from build123d import *

# Parameters (mm, degrees)
SKETCH3_W           = 30
SKETCH3_H           = 30
BOSS_EXTRUDE2_DEPTH = 5
SKETCH4_W           = 22
SKETCH4_H           = 22
BOSS_EXTRUDE3_DEPTH = 3
SKETCH10_R          = 1.5
CUT_EXTRUDE2_DEPTH  = 23.671568098
BOSS_EXTRUDE4_DEPTH = 2.5
SKETCH13_W          = 20
SKETCH13_H          = 3
BOSS_EXTRUDE6_DEPTH = 7.5
FILLET1_R           = 5
MIRROR2_START       = 223.674571743
MIRROR2_OUTLINE_W   = 20
MIRROR2_OUTLINE_H   = 15
MIRROR2_DEPTH       = 3
FILLET2_R           = 5


# Read off the part's stored shape, not the designer's step: Loft-Thin2, Mirror2
with BuildPart() as part:
    # Sketch3 → Boss-Extrude2 (new body)
    with BuildSketch(Plane(origin=(0, 0, 0), x_dir=(1, 0, 0), z_dir=(0, 1, 0))):
        Rectangle(SKETCH3_W, SKETCH3_H)
    extrude(amount=BOSS_EXTRUDE2_DEPTH)

    # Sketch4 → Boss-Extrude3 (add)
    with BuildSketch(Plane(origin=(0, 5, 0), x_dir=(1, 0, 0), z_dir=(0, 1, 0))):
        Rectangle(SKETCH4_W, SKETCH4_H)
    extrude(amount=BOSS_EXTRUDE3_DEPTH)

    # Sketch10 → Cut-Extrude2 (cut, through all)
    with BuildSketch(Plane(origin=(0, 8, 0), x_dir=(1, 0, 0), z_dir=(0, 1, 0))):
        with Locations(Location((-7.071067812, -7.071067812, 0), (0, 0, 270))):
            Circle(SKETCH10_R)
        with Locations(Location((-7.071067812, 7.071067812, 0), (0, 0, 270))):
            Circle(SKETCH10_R)
        with Locations(Location((7.071067812, 7.071067812, 0), (0, 0, 270))):
            Circle(SKETCH10_R)
        with Locations(Location((7.071067812, -7.071067812, 0), (0, 0, 270))):
            Circle(SKETCH10_R)
    extrude(amount=-CUT_EXTRUDE2_DEPTH, mode=Mode.SUBTRACT)

    # Loft-Thin2 outline → Loft-Thin2 (revolve)
    with BuildSketch(Plane.XY):
        Polygon((3.5, 208), (1.499775013, 208), (4.499775013, 8), (6.5, 8), align=None)
    revolve(axis=Axis((0, 0, 0), (0, 1, 0)))

    # Sketch11 → Revolve1 (revolve)
    with BuildSketch(Plane.XY, mode=Mode.PRIVATE) as revolve1_sk:
        Polygon((0, 210.463271105), (3.974140239, 210.463271105), (5.018302856, 160.147044177), (4.217794337, 160.147044177), (3.476729187, 208), (0, 208), align=None)
    revolve(revolve1_sk.sketch.rotate(Axis((0, 233.744226316, 0), (0, -1, 0)), 90), axis=Axis((0, 233.744226316, 0), (0, -1, 0)))

    # Sketch12 → Boss-Extrude4 (add, symmetric)
    with BuildSketch(Plane.XY):
        with BuildLine():
            ThreePointArc((4.833910275, 169.032574831), (20.64513273, 208.670761425), (59.999990588, 225.174571743))
            Line((59.999990588, 225.174571743), (60, 226.674571743))
            ThreePointArc((60, 226.674571743), (19.584436851, 209.731465334), (3.333685749, 169.032574831))
            Line((3.333685749, 169.032574831), (4.833910275, 169.032574831))
        make_face()
    boss_extrude4 = extrude(amount=BOSS_EXTRUDE4_DEPTH, both=True)

    # Mirror1: Boss-Extrude4 across plane
    add(boss_extrude4.mirror(Plane(origin=(0, 0, 0), x_dir=(0, 0, 1), z_dir=(1, 0, 0))))


with BuildPart() as boss_extrude6_tool:
    # Sketch13 → Boss-Extrude6 (new, symmetric)
    with BuildSketch(Plane.XY):
        with Locations((70, 225.174571743)):
            Rectangle(SKETCH13_W, SKETCH13_H)
    extrude(amount=BOSS_EXTRUDE6_DEPTH, both=True)


with BuildPart() as part_1:
    add(part.part)


with BuildPart() as part_2:
    # Boss-Extrude6: joined with boss_extrude6_tool
    add(part_1.part.fuse(boss_extrude6_tool.part, tol=0.00001))

    # Fillet1
    fillet1_edges = [part_2.edges().sort_by_distance(p)[0] for p in [
        (60, 225.174571743, -7.5),
        (80, 225.174571743, -7.5),
        (80, 225.174571743, 7.5),
        (60, 225.174571743, 7.5),
    ]]
    fillet(fillet1_edges, radius=FILLET1_R - 0.0001)  # a hair under: the kernel refuses the full size


with BuildPart() as mirror2_tool:
    # Mirror2 outline → Mirror2 (new body)
    with BuildSketch(Plane(origin=(0, 0, 0), x_dir=(1, 0, 0), z_dir=(0, 1, 0)).offset(MIRROR2_START)):
        with Locations((-70, 0)):
            Rectangle(MIRROR2_OUTLINE_W, MIRROR2_OUTLINE_H)
    extrude(amount=MIRROR2_DEPTH)


with BuildPart() as part_3:
    add(part_2.part)


with BuildPart() as part_4:
    # Mirror2: joined with mirror2_tool
    add(part_3.part.fuse(mirror2_tool.part, tol=0.00001))

    # Fillet2
    fillet2_edges = [part_4.edges().sort_by_distance(p)[0] for p in [
        (-60, 225.174571743, -7.5),
        (-80, 225.174571743, -7.5),
        (-60, 225.174571743, 7.5),
        (-80, 225.174571743, 7.5),
    ]]
    fillet(fillet2_edges, radius=FILLET2_R - 0.0001)  # a hair under: the kernel refuses the full size


solid = part_4.part
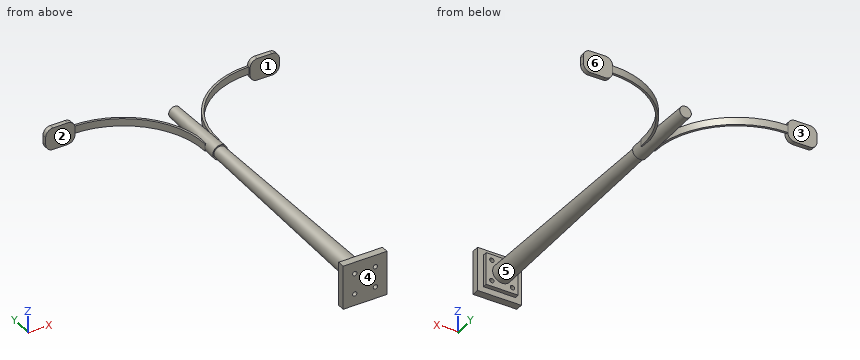
Source: CAD feature listing. Evaluate the final solid. Frame: model axes, mm. Face numbers are marked on the shaded views. A direction names the side the tool comes from. Give positions to 0.01 mm unless a question says otherwise; leave off trailing zeros. Write each loop counter-clockwise with the first axis right and the second up, starting at its lowest first coordinate (ties: lowest second). Pieces come first, ordered by that corner, then holes. Notation, with made-up numbers: (26, 49.25) - (79, 49.25) arc R17 cw to (79, 74.25) - close; hole circle Ø3 at (37.25, 4.25). An arc over 180 degrees is marked (long way). Write item = value, one per line. Start each with the question number.
Q1. Cut plane B-B, the plane x = 68. Return loops of the section in (y, z).
Q2. Cut plane A-A, the plane y = 51. Return loops of the section in (x, z) (3 decimals), then the cut area to 3 significant figures.
Q3. Pin query (flat end, axial travel): pin 1 Ø3 at (y, z) = (157.5, 4.5) entering from +X; pin 2 Ø5 at (x, z) = (22, -1) entering from +Y; pin 3 Ø0.9 at (x, y) = (67.5, 225) entering from -Z. Return the tip coordinate at first contact, or that it passes through.
Q4. Reachability of the marked faces 1, 2 and 3 from +Z, -Z, +X, -X, +Y, -Y: full face, straight path, thin tool, end or side. Return the list, or none.
Q5. Material intervals for probe 1 along Y at (x, z) = (-3.5, 6.5); probe 2 along X at (y, z) = (135, 1.25); probe 3 along X at (y, z) = (29.5, 1.25), sorted ascending.
Q6. Cut plane C-C, the plane x = -24. Return loops of the section in (y, z), then the cut area to 3 significant figures.
Q7. Draft query along Y for the marked faces 4, 5 and 6. Return one class per face: +Y half, -Y half, draft (parallel to the pull), parting line (faces both ways), or undercut.
Q8. Cut plane D-D, the plane y = 24.5. Return loops of the section in (x, z) (1 decimal).
Computed values:
q1.outline = (223.67, -7.5) - (226.67, -7.5) - (226.67, 7.5) - (223.67, 7.5) - close
q2.outline = circle Ø11.71 at (0, 0); hole circle Ø7.71 at (0, 0)
q2.area = 61.0 mm²
q3.pin_1 = 3.02
q3.pin_2 = 214.18
q3.pin_3 = -7.5
q4.face_1 = +Z, -Z, +X, -Y
q4.face_2 = +Z, -Z, -X, -Y
q4.face_3 = +Z, -Z, +X, -X, +Y
q5.probe_1 = 0 to 8
q5.probe_2 = -4.42 to -2.27, 2.27 to 4.42
q5.probe_3 = -6.05 to -3.99, 3.99 to 6.05
q6.outline = (211.81, -2.5) - (213.77, -2.5) - (213.77, 2.5) - (211.81, 2.5) - close
q6.area = 9.80 mm²
q7.face_4 = -Y half
q7.face_5 = undercut
q7.face_6 = +Y half
q8.outline = circle Ø12.5 at (0, 0); hole circle Ø8.5 at (0, 0)
